```python
from build123d import *

# Parameters (mm, degrees)
F0_W     = 81.28
F0_H     = 81.28
F1_DEPTH = 12.7
F2_R     = 28.575
F2_R_2   = 22.225
F3_DEPTH = 53.34
F4_R     = 3.175
F5_DEPTH = 12.701
F6_R     = 6.35
F7_SIZE  = 2.032


with BuildPart() as f1:
    # F0 (on Top) → F1 (new body)
    with BuildSketch(Plane.XY):
        Rectangle(F0_W, F0_H)
    extrude(amount=F1_DEPTH)

    # F2 (on face) → F3 (join)
    with BuildSketch(Plane.XY.offset(12.7)):
        Circle(F2_R)
        Circle(F2_R_2, mode=Mode.SUBTRACT)
    extrude(amount=F3_DEPTH)

    # F4 (on face) → F5 (cut, through all)
    with BuildSketch(Plane.XY.offset(12.7)):
        with Locations((33.02, 33.02)):
            Circle(F4_R)
        with Locations((33.02, -33.02)):
            Circle(F4_R)
        with Locations((-33.02, -33.02)):
            Circle(F4_R)
        with Locations((-33.02, 33.02)):
            Circle(F4_R)
    extrude(amount=-F5_DEPTH, mode=Mode.SUBTRACT)

    # F6
    f6_edges = [f1.edges().sort_by_distance(p)[0] for p in [
        (-40.64, -40.64, 6.35),
        (-40.64, 40.64, 6.35),
        (40.64, 40.64, 6.35),
        (40.64, -40.64, 6.35),
    ]]
    fillet(f6_edges, radius=F6_R)

    # F7
    f7_edges = [f1.edges().sort_by_distance(p)[0] for p in [
        (-22.225, 0, 66.04),
        (-28.575, 0, 66.04),
    ]]
    chamfer(f7_edges, length=F7_SIZE)


solid = f1.part
```
Geometry: final body of the model. Coordinates: model frame, mm. A direction names the side the tool comes from. Coordinates: 2 decimals unless noted, no trailing zeros. Order: outer loops, then holes, each group sorted by start corner. A loop starts at its lowest first (then second) coordinate and runs counter-clockwise, first axis right, second up. Notation, with made-up numbers: (59, 78) -> (78, 78) arc R36 ccw to (78, 117) -> close; hole circle Ø1 at (-7.5, 78.5). An arc over 180 degrees is marked (long way). Use CSV: the item, a comma, the result in double quotes.
1) Section A-A on x = -33.02. Output: boundary loops of the cut face in (y, z) (3 decimals).
Findings:
outline,"(-40.64, 0) -> (-36.195, 0) -> (-36.195, 12.7) -> (-40.64, 12.7) -> close; (-29.845, 0) -> (29.845, 0) -> (29.845, 12.7) -> (-29.845, 12.7) -> close; (36.195, 0) -> (40.64, 0) -> (40.64, 12.7) -> (36.195, 12.7) -> close"
2) Section D-D on z = 51. Output: boundary loops of the cut face in (x, y) (3 decimals).
Findings:
outline,"circle Ø57.15 at (0, 0); hole circle Ø44.45 at (0, 0)"
3) Section C-C on y = 0. Output: boundary loops of the cut face in (x, z) (3 decimals).
Findings:
outline,"(-40.64, 0) -> (40.64, 0) -> (40.64, 12.7) -> (28.575, 12.7) -> (28.575, 64.008) -> (26.543, 66.04) -> (24.257, 66.04) -> (22.225, 64.008) -> (22.225, 12.7) -> (-22.225, 12.7) -> (-22.225, 64.008) -> (-24.257, 66.04) -> (-26.543, 66.04) -> (-28.575, 64.008) -> (-28.575, 12.7) -> (-40.64, 12.7) -> close"
4) Access query for faces 4 (the flat face through (0, 0, 12.7)), 5 (the flat face through (12, -22, 66.04)). Directions: +Z, -Z, +X, -X, +Y, -Y. A direction counts if a zero-diameter tool reaches every point of the face in a straight line with its end or side. Return the directions, or none.
Findings:
face 4,"+Z"
face 5,"+Z, +X, -X, +Y, -Y"
5) Pin query (flat end, axial travel): pin 1 Ø10 at (x, y) = (-33.02, 33.02) entering from -Z; pin 2 Ø10 at (x, y) = (-31.5, -16.5) entering from +Z; pin 3 Ø3 at (x, z) = (27, 56.5) entering from -Y (3 decimals); pin 4 Ø1.5 at (x, y) = (-21.5, 3) entering from +Z. Return the tip coordinate at first contact, or that it passes through.
Findings:
pin 1,"stops at z = 0"
pin 2,"stops at z = 12.7"
pin 3,"stops at y = -12.895"
pin 4,"stops at z = 64.24"
6) Mould query, pull axis X, two halves, no side actions, for faces 1 (the flat face through (40.64, 0, 6)), 2 (the flat face through (-1, 1, 0)), 3 (the cylindrical face through (30.5, 31.09, 6.44)). Classes: +X half, -X half, draft (parallel to the pull), parting line (faces both ways), or undercut.
Findings:
face 1,"+X half"
face 2,"draft"
face 3,"undercut"
7) Line query: line 1 (Y direction, x = 33, z = 9); line 2 (Y direction, x = 0, z = 59) (3 decimals). Output: solid intervals per line, ascending.
Findings:
line 1,"y = -40.64 to -36.19, -29.85 to 29.85, 36.19 to 40.64"
line 2,"y = -28.575 to -22.225, 22.225 to 28.575"
